The listing builds one solid part. Answer for the finished solid, in the listing's coordinates (mm). Face numbers are marked on the shaded views. A direction names the side the tool comes from. Coordinates: 2 decimals unless noted, no trailing zeros. Order: outer loops, then holes, each group sorted by start corner. A loop starts at its lowest first (then second) coordinate and runs counter-clockwise, first axis right, second up.
```python
from build123d import *


with BuildPart() as part:
    # BodySke → Body (revolve)
    with BuildSketch(Plane.XY, mode=Mode.PRIVATE) as body_sk:
        Polygon((2.6924, 0), (3.175, 0), (3.175, 0.53848), (2.42316, 0.53848), (2.42316, 1.103884), (2.6924, 1.103884), (2.6924, 9.268367805), (2.2479, 9.525), (1.2573, 9.525), (1.2573, 11.2522), (2.078566667, 11.2522), (2.2479, 11.421533333), (2.2479, 11.7602), (1.7399, 12.2682), (0, 12.2682), (0, 0.00508), (2.6924, 0.00508), align=None)
    revolve(body_sk.sketch.rotate(Axis((0, 0, 0), (0, 1, 0)), 90), axis=Axis((0, 0, 0), (0, 1, 0)))


solid = part.part
```
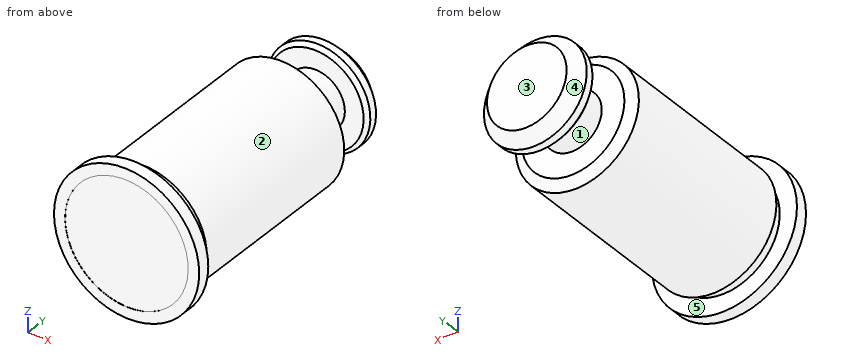
1) This flat-tipped pin is pushed along its axis until it touches: P1, Ø2.5, axis at x = -0.5, z = -0.5, coming from the -Y side. Where does it stop, or does it pass through?
2) A cutting plane is placed at C-C, the plane y = 8. Write down the section's boundary in (x, z), plus the area to 3 significant figures.
3) For the marked faces 4 and 5, determine the directions among +Z, -Z, +X, -X, +Y, -Y from which every point of the face is accessible in a straight line to the end or side of a thin tool.
4) A cutting plane is placed at D-D, the plane x = 3. Write down the section's boundary in (y, z).
5) The mould has two halves that part along Y. Classify the marked faces 1, 2 and 3: released by +Y, released by -Y, zero draft, split by the parting line, or undercut.
6) Straight lines are drawn through the part: probe 1 along Y at (x, z) = (1.5, 0.75) (3 decimals); probe 2 along Y at (x, z) = (-2.5, 1.75); probe 3 along Y at (x, z) = (-0.75, -2) (3 decimals). For each, find the intervals that lie inside material, in ascending order.
Working result:
1. P1: stops at y = 0.01
2. outline: circle Ø5.38 at (0, 0)
2. area: 22.8 mm2
3. face 4: +Y
3. face 5: none
4. outline: (0, -1.04) - (0.54, -1.04) - (0.54, 1.04) - (0, 1.04) - close
5. face 1: undercut
5. face 2: zero draft
5. face 3: released by +Y
6. probe 1: y = 0.005 to 9.525, 11.252 to 12.268
6. probe 2: y = 0 to 0.54
6. probe 3: y = 0.005 to 9.525, 11.31 to 11.872
